Geometry check sheet. Reference: the model listing, model coordinates, mm. A direction names the side the tool comes from. Coordinates: 2 decimals unless noted, no trailing zeros. Loops run counter-clockwise (first coordinate to the right, second up) from the corner with the lowest first, then second, coordinate; pieces in that order, holes last. Notation, with made-up numbers: M -38.75,-6.5 L -28.75,-6.5 A5 cw -28.75,-2.5 Z; hole C -13.75,-15 d9. An arc over 180 degrees is marked long. Use CSV: the item, a comma, the result in double quotes.
```python
from build123d import *

# Parameters (mm, degrees)
F0_W     = 79.95
F0_H     = 19.95
F0_W_2   = 77.95
F0_H_2   = 17.95
F1_DEPTH = 4
F0_W_3   = 83.95
F0_H_3   = 23.95
F2_DEPTH = 1
F4_DEPTH = 100


with BuildPart() as f1:
    # F0 (on Top) → F1 (new body)
    with BuildSketch(Plane.XY):
        Rectangle(F0_W, F0_H)
        Rectangle(F0_W_2, F0_H_2, mode=Mode.SUBTRACT)
    extrude(amount=F1_DEPTH)

    # F0 (on Top) → F2 (join)
    with BuildSketch(Plane.XY):
        Rectangle(F0_W_3, F0_H_3)
        Rectangle(F0_W, F0_H, mode=Mode.SUBTRACT)
        Rectangle(F0_W_2, F0_H_2)
    extrude(amount=F2_DEPTH)

    # F3 (on face) → F4 (cut)
    with BuildSketch(Plane.YZ.offset(39.975)):
        with BuildLine():
            Line((-1.999556, 4), (-1.999556, 3.04214))
            Line((-1.999556, 3.04214), (-1.999556, 2.95786))
            ThreePointArc((-1.999556, 2.95786), (-1.399236, 1.570965), (0, 1))
            ThreePointArc((0, 1), (1.39965, 1.571372), (1.99958, 2.959021))
            Line((1.99958, 2.959021), (1.99958, 3.040979))
            Line((1.99958, 3.040979), (1.99958, 4))
            Line((1.99958, 4), (-1.999556, 4))
        make_face()
    extrude(amount=-F4_DEPTH, mode=Mode.SUBTRACT)


solid = f1.part
```
1. Release check for a two-part mould opening along Y. For faces 5 (the flat face through (-1, -8.975, 2)), 6 (the flat face through (-1, -9.975, 2)), 7 (the flat face through (-39.975, -6, 2)), 8 (the flat face through (-1, 9.975, 2)) record: +Y half, -Y half, draft (parallel to the pull), parting line (faces both ways), or undercut.
The answers:
face 5,"undercut"
face 6,"-Y half"
face 7,"draft"
face 8,"+Y half"
2. Section check B-B, the plane y = 6.25. Record the cut outline in (x, z) (3 decimals), plus the area to 4 significant figures.
The answers:
outline,"M -41.975,0 L 41.975,0 L 41.975,1 L 39.975,1 L 39.975,4 L 38.975,4 L 38.975,1 L -38.975,1 L -38.975,4 L -39.975,4 L -39.975,1 L -41.975,1 Z"
area,"89.95 mm^2"
3. Gauge pin test, flat ends, axial feed: P1, Ø0.9, axis at x = 5, z = 3, coming from the +Y side (3 decimals); P2, Ø1.5, axis at y = 5, z = 3, coming from the -X side (3 decimals); P3, Ø6, axis at x = -13.5, y = -1, coming from the +Z side. Record the tip position at first contact, or that the pin passes through.
The answers:
P1,"y = 9.975"
P2,"x = -39.975"
P3,"z = 1"
4. Thickness scan on line 1 (Y direction, x = 15, z = 2.95) (3 decimals); line 2 (X direction, y = 6.5, z = 2.4) (3 decimals); line 3 (Z direction, x = 5, y = 4). Record the ranges inside material, lowest first. Write a range as [from, to].
The answers:
line 1,"[-9.975, -8.975], [8.975, 9.975]"
line 2,"[-39.975, -38.975], [38.975, 39.975]"
line 3,"[0, 1]"
5. Section check A-A, the plane x = 29.5. Record the cut outline in (y, z) (3 decimals).
The answers:
outline,"M -11.975,0 L 11.975,0 L 11.975,1 L 9.975,1 L 9.975,4 L 8.975,4 L 8.975,1 L -8.975,1 L -8.975,4 L -9.975,4 L -9.975,1 L -11.975,1 Z"
6. Set-up check for faces 1 (the flat face through (39.975, -6, 2)), 2 (the flat face through (-0.2, 9.6, 4)), 3 (the flat face through (-39.975, 6, 2)), 4 (the flat face through (-38.975, -6, 2)): record each of +Z, -Z, +X, -X, +Y, -Y from which the full face is reachable in a straight line by a thin tool's end or side.
The answers:
face 1,"+Z, +X, +Y, -Y"
face 2,"+Z, +X, -X, +Y, -Y"
face 3,"+Z, -X, +Y, -Y"
face 4,"+Z"
